The listing builds one solid part. Answer for the finished solid, in the listing's coordinates (mm). Give positions to 0.01 mm unless a question says otherwise; leave off trailing zeros. Order: outer loops, then holes, each group sorted by start corner. A loop starts at its lowest first (then second) coordinate and runs counter-clockwise, first axis right, second up. Notation, with made-up numbers: (-39, -31) - (-15, -31) arc R32 ccw to (-15, -3) - close; hole circle Ø1 at (32.5, 71.25). An arc over 180 degrees is marked (long way). Write each question's results on one line, items separated by ' | '. Start each with the question number.
1. Flat-ended cylindrical pins translate along their axes: pin 1 (4 mm diameter, centred on x = -314.73, y = 278.51, fed in from +Z); pin 2 (1 mm diameter, centred on y = 274, z = 1, fed in from -X); pin 3 (1 mm diameter, centred on x = -259, z = 0.5, fed in from -Y). Find the tip coordinate at first contact, or state that the pin passes through.
2. Section C-C (x = 294) is taken. Give the vertices of the cut face in (y, z).
3. Section B-B (z = 0.9) is taken. State how many separate pieces and enclosed holes the cut face has, and give its area (3 significant figures).
4. Section A-A (y = 21.5) is taken. Give the vertices of the cut face in (x, z).
5. Find the intervals of material crossed by L1, parallel to Y at x = -60, z = 1.05; L2, parallel to X at y = 7, z = 0.2; L3, parallel to Y at x = -84, z = 1.15, in increasing order.
Solid Edge part; units mm, degrees
sketch "Sketch1" plane through (0, 0, 0) normal (0, 0, 1) x (1, 0, 0)
  line L0 (-183.0017, -120) -> (-227.4217, -120)
  line L1 (-289.5811, -57.8353) -> (-227.4217, -120)
  line L2 (-289.5811, -57.8353) -> (-351.7458, 4.3295)
  line L3 (-351.7458, 129.7437) -> (-351.7458, 4.3295)
  line L4 (-351.7458, 129.7437) -> (-351.7458, 255.1579)
  line L5 (-289.4346, 317.4691) -> (-351.7458, 255.1579)
  line L6 (-289.4346, 317.4691) -> (-227.7006, 379.2031)
  line L7 (0, 379.2031) -> (-227.7006, 379.2031)
  line L8 (0, 379.2031) -> (0, 0)
  line L9 (0, 0) -> (-183.0017, 0)
  line L10 (-183.0017, 0) -> (-183.0017, -120)
  dimension "D1" = 183.0017
  dimension "D2" = 183.0017
  dimension "D3" = 289.4346
  dimension "D4" = 289.4346
  dimension "D5" = 351.7458
  dimension "D6" = 351.7458
  dimension "D7" = 289.5811
  dimension "D8" = 289.5811
extrude "Protrusion1" add sketch "Sketch1" along normal blind 3
mirror "Mirror1" about plane through (0, 0, 0) normal (1, 0, 0) of "Protrusion1"
sketch "Sketch2" plane through (0, 149.6016, 0) normal (0, 0, -1) x (-1, 0, 0)
  line L0 (-351.7458, -111.1142) -> (-193.1203, -269.6016)
  line L1 (-193.1203, -269.6016) -> (-227.4217, -269.6016)
  arc A0 (-351.7458, -145.2721) -> (-227.4217, -269.6016) centre (-220.2414, -138.0974) ccw
  line L2 (-351.7458, -111.1142) -> (-351.7458, -145.2721)
extrude "Protrusion2" add sketch "Sketch2" against normal up to vertex (3 mm away)
sketch "Sketch3" plane through (0, 149.6016, 0) normal (0, 0, -1) x (-1, 0, 0)
  line L0 (-227.7006, 229.6016) -> (-351.7458, 105.5563)
  arc A0 (-351.7458, 105.5563) -> (-227.7006, 229.6016) centre (-220.2564, 98.1121) cw
extrude "Protrusion3" add sketch "Sketch3" against normal up to vertex (3 mm away)
mirror "Mirror2" about plane through (0, 0, 0) normal (1, 0, 0) of "Protrusion3", "Protrusion2"
sketch "Sketch4" plane through (0, 0, 2.5) normal (0, -1, 0) x (1, 0, 0)
  line L0 (-183.0017, 0.5) -> (183.0017, 0.5)
  line L1 (183.0017, 0.5) -> (183.0017, -2.5)
  line L2 (183.0017, -2.5) -> (-183.0017, -2.5)
  line L3 (-183.0017, -2.5) -> (-183.0017, 0.5)
extrude "Protrusion6" add sketch "Sketch4" along normal blind 1.13
sketch "Sketch5" plane through (0, 129.6016, 3) normal (0, 0, 1) x (1, 0, 0)
  line L0 (-183.0017, -130.7316) -> (183.0017, -130.7316)
  line L1 (183.0017, -130.7316) -> (183.0017, -115.7316)
  line L2 (183.0017, -115.7316) -> (-183.0017, -115.7316)
  line L3 (-183.0017, -115.7316) -> (-183.0017, -130.7316)
  dimension "D1" = 183.0017
extrude "Cutout1" cut sketch "Sketch5" against normal through all
sketch "Sketch6" plane through (0, 129.6016, 3) normal (0, 0, 1) x (1, 0, 0)
  circle A0 centre (-203.0017, -232.7016) radius 3.5
  circle A1 centre (203.0017, -232.7016) radius 3.5
extrude "Cutout2" cut sketch "Sketch6" against normal through all
sketch "Sketch7" plane through (0, 129.6016, 3) normal (0, 0, 1) x (1, 0, 0)
  circle A0 centre (-60, 219.6016) radius 3.5
  circle A1 centre (60, 219.6016) radius 3.5
extrude "Cutout3" cut sketch "Sketch7" against normal through all
sketch "Sketch8" plane through (0, 129.6016, 3) normal (0, 0, 1) x (1, 0, 0)
  line L0 (-351.7458, 125.5563) -> (-227.7006, 249.6016)
  line L1 (-227.7006, 249.6016) -> (-363.4952, 305.1732)
  line L2 (-363.4952, 305.1732) -> (-448.4916, 154.169)
  line L3 (-448.4916, 154.169) -> (-351.7458, 125.5563)
  line L4 (227.7006, 249.6016) -> (351.7458, 125.5563)
  line L5 (451.8618, 235.0605) -> (351.7458, 125.5563)
  line L6 (265.8398, 326.8744) -> (451.8618, 235.0605)
  line L7 (227.7006, 249.6016) -> (265.8398, 326.8744)
  line L8 (-351.7458, -125.2721) -> (-227.4217, -249.6016)
  line L9 (-294.7747, -355.8094) -> (-227.4217, -249.6016)
  line L10 (-435.8326, -227.4106) -> (-294.7747, -355.8094)
  line L11 (-351.7458, -125.2721) -> (-435.8326, -227.4106)
  line L12 (227.4217, -249.6016) -> (351.7458, -125.2721)
  line L13 (351.7458, -125.2721) -> (481.0434, -232.7016)
  line L14 (481.0434, -232.7016) -> (340.8898, -317.8323)
  line L15 (340.8898, -317.8323) -> (227.4217, -249.6016)
extrude "Cutout4" cut sketch "Sketch8" against normal through all
sketch "Sketch9" plane through (0, 129.6016, 3) normal (0, 0, 1) x (1, 0, 0)
  line L0 (-241.9037, 279.2919) -> (241.9037, 279.2919)
  line L1 (241.9037, 279.2919) -> (241.9037, 235.3984)
  line L2 (241.9037, 235.3984) -> (-241.9037, 235.3984)
  line L3 (-241.9037, 235.3984) -> (-241.9037, 279.2919)
extrude "Cutout5" cut sketch "Sketch9" against normal through all
sketch "Sketch10" plane through (0, 122.5, 3) normal (0, 0, 1) x (1, 0, 0)
  circle A0 centre (-314.7299, 156.0117) radius 3.5
  circle A1 centre (-152, 226.7031) radius 3.5
  circle A2 centre (152, 226.7031) radius 3.5
  circle A3 centre (244, 226.7031) radius 3.5
  circle A4 centre (314.7107, 155.9924) radius 3.5
  circle A5 centre (-244, 226.7031) radius 3.5
  dimension "D1" = 314.7299
  dimension "D2" = 244
extrude "Cutout6" cut sketch "Sketch10" against normal through all
sketch "Sketch11" plane through (0, 122.5, 3) normal (0, 0, 1) x (1, 0, 0)
  line L0 (-346.7458, -123.1707) -> (-389.0462, -123.1707)
  line L1 (-389.0462, -123.1707) -> (-389.0462, 137.6579)
  line L2 (-389.0462, 137.6579) -> (-346.7458, 137.6579)
  line L3 (-346.7458, 137.6579) -> (-346.7458, -123.1707)
  line L4 (346.7458, -123.1707) -> (391.6035, -123.1707)
  line L5 (391.6035, -123.1707) -> (391.6035, 137.6579)
  line L6 (391.6035, 137.6579) -> (346.7458, 137.6579)
  line L7 (346.7458, 137.6579) -> (346.7458, -123.1707)
extrude "Cutout7" cut sketch "Sketch11" against normal through all
sketch "Sketch12" plane through (0, 122.5, 3) normal (0, 0, 1) x (1, 0, 0)
  line L0 (-183.0017, -108.63) -> (183.0017, -108.63)
  line L1 (183.0017, -108.63) -> (183.0017, -84.5)
  line L2 (183.0017, -84.5) -> (-183.0017, -84.5)
  line L3 (-183.0017, -84.5) -> (-183.0017, -108.63)
extrude "Cutout8" cut sketch "Sketch12" against normal through all
sketch "Sketch13" plane through (0, 122.5, 3) normal (0, 0, 1) x (1, 0, 0)
  line L0 (-227.4217, -242.5) -> (-346.7458, -138.1707)
  line L1 (-346.7458, -138.1707) -> (-346.7458, -123.1707)
  line L2 (-346.7458, -123.1707) -> (-227.4217, -242.5)
  line L3 (227.4217, -242.5) -> (346.7458, -123.1707)
  line L4 (346.7458, -123.1707) -> (346.7458, -138.1707)
  line L5 (346.7458, -138.1707) -> (227.4217, -242.5)
  dimension "D1" = 346.7458
  dimension "D2" = 346.7458
extrude "Protrusion7" add sketch "Sketch13" against normal up to vertex (3 mm away)
sketch "Sketch14" plane through (0, 122.5, 3) normal (0, 0, 1) x (1, 0, 0)
  line L0 (-241.7458, 242.5) -> (-346.7458, 137.5)
  line L1 (-346.7458, 137.5) -> (-371.6237, 169.0493)
  line L2 (-371.6237, 169.0493) -> (-268.0776, 273.8459)
  line L3 (-268.0776, 273.8459) -> (-241.7458, 242.5)
extrude "Cutout9" cut sketch "Sketch14" against normal through all
mirror "Mirror3" about plane through (0, 0, 0) normal (1, 0, 0) of "Cutout9"
sketch "Sketch15" plane through (0, 122.5, 3) normal (0, 0, 1) x (1, 0, 0)
  line L0 (-226.7458, -242.5) -> (-346.7458, -137.5)
  line L1 (-346.7458, -137.5) -> (-366.1295, -195.1398)
  line L2 (-366.1295, -195.1398) -> (-252.7979, -291.374)
  line L3 (-252.7979, -291.374) -> (-226.7458, -242.5)
extrude "Cutout10" cut sketch "Sketch15" against normal through all
mirror "Mirror4" about plane through (0, 0, 0) normal (1, 0, 0) of "Cutout10"
properties material "ABS-Plastik, mittelfest"
Reported:
1) pin 1: through | pin 2: x = -333.25 | pin 3: y = -92.22
2) outline: (-61.15, 0) - (312.75, 0) - (312.75, 3) - (-61.15, 3) - close
3) separate pieces: 1 | enclosed holes: 10 | area: 255,000 mm²
4) outline: (-346.75, 0) - (-183, 0) - (-183, 3) - (-346.75, 3) - close; (183, 0) - (346.75, 0) - (346.75, 3) - (183, 3) - close
5) L1: 38 to 345.7, 352.7 to 365 | L2: -346.75 to -183, 183 to 346.75 | L3: 38 to 365
